```python
from build123d import *

# Parameters (mm, degrees)
SKETCH_1_W               = 31.1
SKETCH_1_H               = 31.1
SKETCH_1_W_2             = 21.1
SKETCH_1_H_2             = 21.1
EXTRUDE_1_DEPTH          = 60
SKETCH_2_R               = 1.55
CUT_EXTRUDE_1_DEPTH      = 73.445979875
CUT_EXTRUDE_2_DEPTH      = 71.444446197
CUT_EXTRUDE_2_DEPTH_BACK = 71.444446197
SKETCH_3_W               = 2.7
SKETCH_3_H               = 6
SKETCH_4_R               = 1.55
CUT_EXTRUDE_3_DEPTH      = 73.445979875
CUT_EXTRUDE_4_DEPTH      = 71.444446197
CUT_EXTRUDE_4_DEPTH_BACK = 71.444446197
SKETCH_5_W               = 3.5
SKETCH_5_H               = 6.2
FILLET_1_R               = 1.5
SKETCH_6_W               = 20.2
SKETCH_6_H               = 20.2
CUT_EXTRUDE_5_DEPTH      = 73.445979875
SKETCH_7_R               = 1.55
EXTRUDE_2_DEPTH          = 2.25
EXTRUDE_START            = 2.25
SKETCH_8_R               = 1.55
EXTRUDE_3_DEPTH          = 2.25
SKETCH_9_W               = 5
SKETCH_9_H               = 60
CUT_EXTRUDE_6_DEPTH      = 75.488723979


with BuildPart() as part:
    # 草图1 → 凸台-拉伸1 (new body)
    with BuildSketch(Plane(origin=(0, 0, 0), x_dir=(1, 0, 0), z_dir=(0, 1, 0))):
        with Locations((10.55, 10.55)):
            Rectangle(SKETCH_1_W, SKETCH_1_H)
        with Locations((10.55, 10.55)):
            Rectangle(SKETCH_1_W_2, SKETCH_1_H_2, mode=Mode.SUBTRACT)
    extrude(amount=EXTRUDE_1_DEPTH)

    # 草图2 → 切除-拉伸1 (cut, through all)
    with BuildSketch(Plane.ZY.offset(5)):
        with Locations((-23.6, 57)):
            Circle(SKETCH_2_R)
        with Locations((-23.6, 3)):
            Circle(SKETCH_2_R)
        with Locations((2.5, 3)):
            Circle(SKETCH_2_R)
        with Locations((2.5, 57)):
            Circle(SKETCH_2_R)
    extrude(amount=-CUT_EXTRUDE_1_DEPTH, mode=Mode.SUBTRACT)

    # 草图3 → 切除-拉伸2 (cut, two sides: drawn at the far end of the back side and taken through both)
    with BuildSketch(Plane.XY.offset(-21.1).offset(-CUT_EXTRUDE_2_DEPTH_BACK)):
        with Locations((6.2, 57)):
            Rectangle(SKETCH_3_W, SKETCH_3_H)
        with Locations((14.9, 57)):
            Rectangle(SKETCH_3_W, SKETCH_3_H)
        with Locations((14.9, 3)):
            Rectangle(SKETCH_3_W, SKETCH_3_H)
        with Locations((6.2, 3)):
            Rectangle(SKETCH_3_W, SKETCH_3_H)
    extrude(amount=CUT_EXTRUDE_2_DEPTH + CUT_EXTRUDE_2_DEPTH_BACK, mode=Mode.SUBTRACT)

    # 草图4 → 切除-拉伸3 (cut, through all)
    with BuildSketch(Plane(origin=(0, 0, -26.1), x_dir=(-1, 0, 0), z_dir=(0, 0, -1))):
        with Locations((-23.6, 53)):
            Circle(SKETCH_4_R)
        with Locations((2.5, 53)):
            Circle(SKETCH_4_R)
        with Locations((2.5, 7)):
            Circle(SKETCH_4_R)
        with Locations((-23.6, 7)):
            Circle(SKETCH_4_R)
    extrude(amount=-CUT_EXTRUDE_3_DEPTH, mode=Mode.SUBTRACT)

    # 草图5 → 切除-拉伸4 (cut, two sides: drawn at the far end of the back side and taken through both)
    with BuildSketch(Plane.ZY.offset(-21.1).offset(-CUT_EXTRUDE_4_DEPTH_BACK)):
        with Locations((-15.3, 53)):
            Rectangle(SKETCH_5_W, SKETCH_5_H)
        with Locations((-5.8, 53)):
            Rectangle(SKETCH_5_W, SKETCH_5_H)
        with Locations((-5.8, 7)):
            Rectangle(SKETCH_5_W, SKETCH_5_H)
        with Locations((-15.3, 7)):
            Rectangle(SKETCH_5_W, SKETCH_5_H)
    extrude(amount=CUT_EXTRUDE_4_DEPTH + CUT_EXTRUDE_4_DEPTH_BACK, mode=Mode.SUBTRACT)

    # 圆角1
    fillet_1_edges = [part.edges().sort_by_distance(p)[0] for p in [
        (14.9, 6, 0),
        (14.9, 6, -26.1),
        (14.9, 6, 5),
        (14.9, 54, 0),
        (14.9, 54, -26.1),
        (14.9, 54, 5),
        (6.2, 54, 0),
        (6.2, 54, -26.1),
        (6.2, 54, 5),
        (21.1, 49.9, -15.3),
        (21.1, 56.1, -15.3),
        (21.1, 49.9, -5.8),
        (21.1, 56.1, -5.8),
        (21.1, 10.1, -5.8),
        (21.1, 3.9, -5.8),
        (21.1, 10.1, -15.3),
        (21.1, 3.9, -15.3),
        (0, 3.9, -15.3),
        (0, 10.1, -15.3),
        (26.1, 3.9, -15.3),
        (26.1, 10.1, -15.3),
        (-5, 3.9, -15.3),
        (-5, 10.1, -15.3),
        (0, 3.9, -5.8),
        (0, 10.1, -5.8),
        (26.1, 3.9, -5.8),
        (26.1, 10.1, -5.8),
        (-5, 3.9, -5.8),
        (-5, 10.1, -5.8),
        (0, 56.1, -5.8),
        (0, 49.9, -5.8),
        (26.1, 56.1, -5.8),
        (26.1, 49.9, -5.8),
        (-5, 49.9, -5.8),
        (-5, 56.1, -5.8),
        (0, 56.1, -15.3),
        (0, 49.9, -15.3),
        (26.1, 56.1, -15.3),
        (26.1, 49.9, -15.3),
        (-5, 49.9, -15.3),
        (-5, 56.1, -15.3),
        (6.2, 54, -21.1),
        (14.9, 54, -21.1),
        (14.9, 6, -21.1),
        (6.2, 6, -21.1),
        (6.2, 6, 0),
        (6.2, 6, -26.1),
        (6.2, 6, 5),
    ]]
    fillet(fillet_1_edges, radius=FILLET_1_R)

    # 草图6 → 切除-拉伸5 (cut, through all)
    with BuildSketch(Plane.XY.offset(5)):
        with Locations((10.55, 30)):
            Rectangle(SKETCH_6_W, SKETCH_6_H)
    extrude(amount=-CUT_EXTRUDE_5_DEPTH, mode=Mode.SUBTRACT)

    # 草图7 → 凸台-拉伸2 (add)
    with BuildSketch(Plane.XY.offset(5)):
        Polygon((13.55, 0), (13.55, 7.5), (16.25, 7.5), (16.25, 0), (26.1, 0), (26.1, 60), (16.25, 60), (16.25, 52.5), (13.55, 52.5), (13.55, 60), (7.55, 60), (7.55, 52.5), (4.85, 52.5), (4.85, 60), (-5, 60), (-5, 0), (4.85, 0), (4.85, 7.5), (7.55, 7.5), (7.55, 0), align=None)
        with Locations(Location((23.6, 7, 0), (0, 0, 180))):
            Circle(SKETCH_7_R, mode=Mode.SUBTRACT)
        with Locations(Location((23.6, 53, 0), (0, 0, 180))):
            Circle(SKETCH_7_R, mode=Mode.SUBTRACT)
        with Locations(Location((-2.5, 53, 0), (0, 0, 180))):
            Circle(SKETCH_7_R, mode=Mode.SUBTRACT)
        with Locations(Location((-2.5, 7, 0), (0, 0, 180))):
            Circle(SKETCH_7_R, mode=Mode.SUBTRACT)
    extrude(amount=EXTRUDE_2_DEPTH)

    # 草图8 → 凸台-拉伸3 (add)
    with BuildSketch(Plane(origin=(0, 0, -26.1), x_dir=(-1, 0, 0), z_dir=(0, 0, -1)).offset(EXTRUDE_START)):
        Polygon((-7.55, 7.5), (-4.85, 7.5), (-4.85, 0), (5, 0), (5, 60), (-4.85, 60), (-4.85, 52.5), (-7.55, 52.5), (-7.55, 60), (-13.55, 60), (-13.55, 52.5), (-16.25, 52.5), (-16.25, 60), (-26.1, 60), (-26.1, 0), (-16.25, 0), (-16.25, 7.5), (-13.55, 7.5), (-13.55, 0), (-7.55, 0), align=None)
        with Locations((-23.6, 7)):
            Circle(SKETCH_8_R, mode=Mode.SUBTRACT)
        with Locations((2.5, 7)):
            Circle(SKETCH_8_R, mode=Mode.SUBTRACT)
        with Locations((2.5, 53)):
            Circle(SKETCH_8_R, mode=Mode.SUBTRACT)
        with Locations((-23.6, 53)):
            Circle(SKETCH_8_R, mode=Mode.SUBTRACT)
    extrude(amount=-EXTRUDE_3_DEPTH)

    # 草图9 → 切除-拉伸6 (cut, through all)
    with BuildSketch(Plane(origin=(0, 0, -28.35), x_dir=(-1, 0, 0), z_dir=(0, 0, -1))):
        with Locations((-23.6, 30)):
            Rectangle(SKETCH_9_W, SKETCH_9_H)
    extrude(amount=-CUT_EXTRUDE_6_DEPTH, mode=Mode.SUBTRACT)


solid = part.part
```
Source: CAD feature listing. Evaluate the final solid. Frame: model axes, mm. A direction names the side the tool comes from. Give positions to 0.01 mm unless a question says otherwise; leave off trailing zeros. Loops run counter-clockwise (first coordinate to the right, second up) from the corner with the lowest first, then second, coordinate; pieces in that order, holes last. Notation, with made-up numbers: (-24.75, -16) -> (23.25, -16) arc R20 ccw to (23.25, 1) -> close; hole circle Ø8 at (-14, -11). An arc over 180 degrees is marked (long way). Use a Markdown table: item, result. Add a question column.
(1) Section query A-A (x = 10.25). Output: boundary loops of the cut face in (y, z), then the cut area to 3 significant figures.
(2) Section query B-B (z = -23.6). Count the separate pieces of the cut face and the enclosed holes in it, then the cut area to 3 significant figures.
(3) Access query for faces 1 (the face through (-4.57, 10.55, -5.82)), 2 (the face through (14.92, 6.45, -25.67)), 3 (the face through (0, 30, -10)), 4 (the face through (6, 52.5, 6)). Directions: +Z, -Z, +X, -X, +Y, -Y. A direction counts if a zero-diameter tool reaches every point of the face in a straight line with its end or side. Return the directions, or none.
(4) Section query D-D (y = 25). Output: boundary loops of the cut face in (x, z), then the cut area to 3 significant figures.
(5) Pull-direction query (X, two-part tool) for faces 5 (the face through (10, 16, 0)), 6 (the face through (10, 19.9, 3)), 7 (the face through (20.65, 30, -24)), 8 (the face through (-0.45, 3.47, -15.32)); classes: +X half, -X half, draft (parallel to the pull), parting line (faces both ways), or undercut.
(6) First-contact query: pin 1 Ø0.7 at (x, z) = (6, 6.5) entering from +Y; pin 2 Ø12 at (x, z) = (10, -9) entering from +Y; pin 3 Ø1 at (y, z) = (50.5, -20) entering from +X; pin 4 Ø0.6 at (x, z) = (14.5, 2.5) entering from -Y. Flat tips, straight axial feed; report the tip coordinate or a pass-through.
(7) Section query C-C (x = 5.75). Output: boundary loops of the cut face in (y, z).
(8) Ray query, line 1 (Z direction, x = -1.5, y = 54.5); line 2 (X direction, y = 55.5, z = -22); line 3 (Y direction, x = 2.25, z = -23.6). Return the intervals inside material, ascending.
Checked values:
| question | item | result |
|---|---|---|
| 1 | outline | (0, -28.35) -> (60, -28.35) -> (60, -21.1) -> (40.1, -21.1) -> (40.1, -26.1) -> (19.9, -26.1) -> (19.9, -21.1) -> (0, -21.1) -> close; (0, 0) -> (19.9, 0) -> (19.9, 5) -> (40.1, 5) -> (40.1, 0) -> (60, 0) -> (60, 7.25) -> (0, 7.25) -> close; hole circle Ø3.1 at (3, -23.6); hole circle Ø3.1 at (3, 2.5); hole circle Ø3.1 at (57, -23.6); hole circle Ø3.1 at (57, 2.5) |
| 1 | area | 638 mm^2 |
| 2 | separate pieces | 7 |
| 2 | enclosed holes | 3 |
| 2 | area | 950 mm^2 |
| 3 | face 1 | -X |
| 3 | face 2 | -Z, -Y |
| 3 | face 3 | +X, +Y, -Y |
| 3 | face 4 | +Z, +Y |
| 4 | outline | (-5, -28.35) -> (21.1, -28.35) -> (21.1, -21.1) -> (20.65, -21.1) -> (20.65, -26.1) -> (0.45, -26.1) -> (0.45, -21.1) -> (0, -21.1) -> (0, 0) -> (0.45, 0) -> (0.45, 5) -> (20.65, 5) -> (20.65, 0) -> (21.1, 0) -> (21.1, 7.25) -> (-5, 7.25) -> close |
| 4 | area | 282 mm^2 |
| 5 | face 5 | draft |
| 5 | face 6 | undercut |
| 5 | face 7 | undercut |
| 5 | face 8 | +X half |
| 6 | pin 1 | y = 52.5 |
| 6 | pin 2 | through |
| 6 | pin 3 | x = 0 |
| 6 | pin 4 | y = 6 |
| 7 | outline | (6, -24.6) arc R1.5 ccw to (7.5, -26.1) -> (7.5, -28.35) -> (52.5, -28.35) -> (52.5, -26.1) arc R1.5 ccw to (54, -24.6) -> (54, -22.6) arc R1.5 ccw to (52.5, -21.1) -> (40.1, -21.1) -> (40.1, -26.1) -> (19.9, -26.1) -> (19.9, -21.1) -> (7.5, -21.1) arc R1.5 ccw to (6, -22.6) -> close; (6, 1.5) arc R1.5 ccw to (7.5, 0) -> (19.9, 0) -> (19.9, 5) -> (40.1, 5) -> (40.1, 0) -> (52.5, 0) arc R1.5 ccw to (54, 1.5) -> (54, 3.5) arc R1.5 ccw to (52.5, 5) -> (52.5, 7.25) -> (7.5, 7.25) -> (7.5, 5) arc R1.5 ccw to (6, 3.5) -> close |
| 8 | line 1 | -28.35 to -17.05, -13.55 to -7.55, -4.05 to 7.25 |
| 8 | line 2 | -5 to 4.85, 7.55 to 13.55, 16.25 to 21.1 |
| 8 | line 3 | 0 to 1.45, 4.55 to 19.9, 40.1 to 55.45, 58.55 to 60 |
